Design review of the part shown in the three views and the two pictorial views. Dimensions are in mm from the part's minimum x, y and z. Round coordinates to 2 decimals unless told otherwise and drop trailing zeros. Write each loop counter-clockwise with the first axis right and the second up, starting at its lowest first coordinate (ties: lowest second). Pieces come first, ordered by that corner, then holes. Notation, with made-up numbers: (-8.75, -15.75) - (17.25, -15.75) arc R13 cw to (17.25, -0.75) - close; hole circle Ø2 at (87, 45). An arc over 180 degrees is marked (long way). Use one line per item in the form item = value.
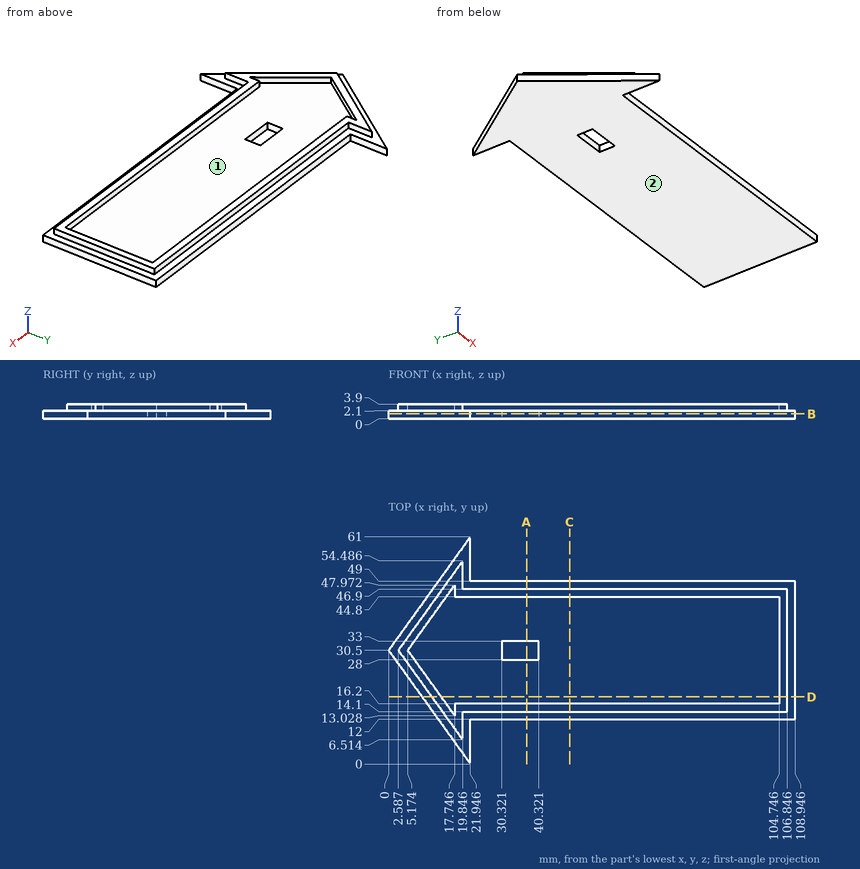
(1) Add section A-A on x = 37. Write out the cut boundary in (y, z).
Geometry results:
outline = (12, 0) - (28, 0) - (28, 2.1) - (16.2, 2.1) - (16.2, 3.9) - (14.1, 3.9) - (14.1, 2.1) - (12, 2.1) - close; (33, 0) - (49, 0) - (49, 2.1) - (46.9, 2.1) - (46.9, 3.9) - (44.8, 3.9) - (44.8, 2.1) - (33, 2.1) - close
(2) The part is to be moulded in two halves that separate along X. For the marked faces 1 and 2, say which applies: +X half, -X half, draft (parallel to the pull), parting line (faces both ways), or undercut.
Geometry results:
face_1 = undercut
face_2 = draft
(3) Add section B-B on z = 1.25. Write out the cut boundary in (x, y), then the cut area to 3 significant figures.
Geometry results:
outline = (0, 30.5) - (21.95, 0) - (21.95, 12) - (108.95, 12) - (108.95, 49) - (21.95, 49) - (21.95, 61) - close; hole (30.32, 28) - (40.32, 28) - (40.32, 33) - (30.32, 33) - close
area = 3,840 mm2
(4) To check wall thickness, follow L1, parallel to Y at x = 51, z = 3.5; L2, parallel to Y at x = 38, z = 1.6; L3, parallel to Z at x = 25.5, y = 29. State the ranges of each line that lie inside material, in increasing order.
Geometry results:
L1 = 14.1 to 16.2, 44.8 to 46.9
L2 = 12 to 28, 33 to 49
L3 = 0 to 2.1
(5) Add section D-D on y = 18. Write out the cut boundary in (x, z).
Geometry results:
outline = (8.99, 0) - (108.95, 0) - (108.95, 2.1) - (106.85, 2.1) - (106.85, 3.9) - (104.75, 3.9) - (104.75, 2.1) - (14.17, 2.1) - (14.17, 3.9) - (11.58, 3.9) - (11.58, 2.1) - (8.99, 2.1) - close
(6) Insertion check: P1, Ø6, axis at x = 33, y = 39.5, coming from the +Z side; P2, Ø0.9, axis at y = 46, z = 3, coming from the -X side; P3, Ø2, axis at x = 66.5, z = 3, coming from the +Y side; P4, Ø1.7, axis at y = 30, z = 1.5, coming from the -X side. Each pin has a flat end and moves straight along its axis. Give the tip position at first contact, or say it passes through.
Geometry results:
P1 = 2.1
P2 = 13.42
P3 = 49
P4 = 0
(7) Add section C-C on x = 48.5. Write out the cut boundary in (y, z).
Geometry results:
outline = (12, 0) - (49, 0) - (49, 2.1) - (46.9, 2.1) - (46.9, 3.9) - (44.8, 3.9) - (44.8, 2.1) - (16.2, 2.1) - (16.2, 3.9) - (14.1, 3.9) - (14.1, 2.1) - (12, 2.1) - close
